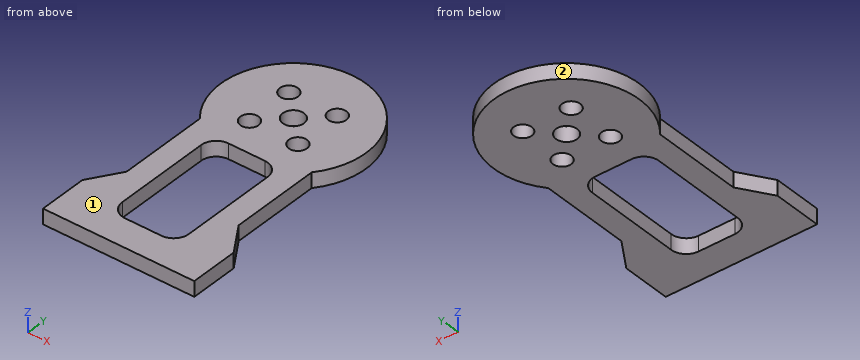
from build123d import *

# Parameters (mm, degrees)
SZKIC1_R                    = 1.75
SZKIC1_R_2                  = 1.5
DODANIE_WYCI_GNI_CIE1_DEPTH = 2.5


with BuildPart() as part:
    # Szkic1 → Dodanie-wyciągnięcie1 (new body)
    with BuildSketch(Plane.XY):
        with BuildLine():
            Line((12.5, 0), (-12.5, 0))
            Line((-12.5, 0), (-12.5, 8))
            Line((-12.5, 8), (-9.25, 13))
            Line((-9.25, 13), (-9.25, 27.855557574))
            ThreePointArc((-9.25, 27.855557574), (0, 47.5), (9.25, 27.855557574))
            Line((9.25, 27.855557574), (9.25, 13))
            Line((9.25, 13), (12.5, 8))
            Line((12.5, 8), (12.5, 0))
        make_face()
        with Locations((0, 35.5)):
            Circle(SZKIC1_R, mode=Mode.SUBTRACT)
        with Locations((-4, 39.5)):
            Circle(SZKIC1_R_2, mode=Mode.SUBTRACT)
        with Locations(Location((-4, 31.5, 0), (0, 0, 180))):
            Circle(SZKIC1_R_2, mode=Mode.SUBTRACT)
        with Locations((4, 31.5)):
            Circle(SZKIC1_R_2, mode=Mode.SUBTRACT)
        with Locations(Location((4, 39.5, 0), (0, 0, 180))):
            Circle(SZKIC1_R_2, mode=Mode.SUBTRACT)
        with BuildLine():
            Line((3, 5), (-3, 5))
            ThreePointArc((-3, 5), (-4.767766953, 5.732233047), (-5.5, 7.5))
            Line((-5.5, 7.5), (-5.5, 23.5))
            ThreePointArc((-5.5, 23.5), (-4.767766953, 25.267766953), (-3, 26))
            Line((-3, 26), (3, 26))
            ThreePointArc((3, 26), (4.767766953, 25.267766953), (5.5, 23.5))
            Line((5.5, 23.5), (5.5, 7.5))
            ThreePointArc((5.5, 7.5), (4.767766953, 5.732233047), (3, 5))
        make_face(mode=Mode.SUBTRACT)
    extrude(amount=DODANIE_WYCI_GNI_CIE1_DEPTH)


solid = part.part
Check sheet for the modelled part. Datum: model origin and axes. Units: mm. Face numbers are marked on the shaded views. Round coordinates to 2 decimals unless told otherwise and drop trailing zeros. Write each loop counter-clockwise with the first axis right and the second up, starting at its lowest first coordinate (ties: lowest second). Pieces come first, ordered by that corner, then holes. Notation, with made-up numbers: (85, 79.5) - (111, 79.5) arc R11 ccw to (111, 91.5) - close; hole circle Ø3 at (38, 25.25). An arc over 180 degrees is marked (long way). Return JSON: item names as keys, results as strings.
Q1. Scan lines: L1, parallel to X at y = 13, z = 1.55; L2, parallel to Y at x = 0, z = 1.55; L3, parallel to Y at x = 4, z = 1.1. Record each from-to range of solid material in increasing order. Write a range as from..to.
Returned:
{"L1": "x = -9.25..-5.5, 5.5..9.25", "L2": "y = 0..5, 26..33.75, 37.25..47.5", "L3": "y = 0..5.21, 25.79..30, 33..38, 41..46.81"}
Q2. Cross-section at B-B (z = 0.95). Record the boundary of the cut face in (x, y).
Returned:
{"outline": "(-12.5, 0) - (12.5, 0) - (12.5, 8) - (9.25, 13) - (9.25, 27.86) arc R12 ccw (long way) to (-9.25, 27.86) - (-9.25, 13) - (-12.5, 8) - close; hole (-5.5, 7.5) arc R2.5 ccw to (-3, 5) - (3, 5) arc R2.5 ccw to (5.5, 7.5) - (5.5, 23.5) arc R2.5 ccw to (3, 26) - (-3, 26) arc R2.5 ccw to (-5.5, 23.5) - close; hole circle Ø3 at (-4, 31.5); hole circle Ø3 at (-4, 39.5); hole circle Ø3.5 at (0, 35.5); hole circle Ø3 at (4, 31.5); hole circle Ø3 at (4, 39.5)"}
Q3. Cross-section at A-A (y = 21). Record the boundary of the cut face in (x, z).
Returned:
{"outline": "(-9.25, 0) - (-5.5, 0) - (-5.5, 2.5) - (-9.25, 2.5) - close; (5.5, 0) - (9.25, 0) - (9.25, 2.5) - (5.5, 2.5) - close"}
Q4. Draft check along Y on the marked faces 1 and 2. Enter one of: released by +Y, released by -Y, zero draft, split by the parting line, or undercut.
Returned:
{"face 1": "zero draft", "face 2": "undercut"}
Q5. Cross-section at D-D (y = 39). Record the boundary of the cut face in (x, z).
Returned:
{"outline": "(-11.48, 0) - (-5.41, 0) - (-5.41, 2.5) - (-11.48, 2.5) - close; (-2.59, 0) - (2.59, 0) - (2.59, 2.5) - (-2.59, 2.5) - close; (5.41, 0) - (11.48, 0) - (11.48, 2.5) - (5.41, 2.5) - close"}
Q6. Depth check by flat-ended pin: P1, Ø1.8, axis at x = 4, y = 39.5, coming from the +Z side; P2, Ø0.8, axis at y = 20.5, z = 1, coming from the +X side. Enter the tip coordinate at first touch or a pass-through.
Returned:
{"P1": "passes through", "P2": "stops at x = 9.25"}
Q7. Cross-section at C-C (x = 0). Record the boundary of the cut face in (y, z), then the cut area to 3 significant figures.
Returned:
{"outline": "(0, 0) - (5, 0) - (5, 2.5) - (0, 2.5) - close; (26, 0) - (33.75, 0) - (33.75, 2.5) - (26, 2.5) - close; (37.25, 0) - (47.5, 0) - (47.5, 2.5) - (37.25, 2.5) - close", "area": "57.5 mm²"}
